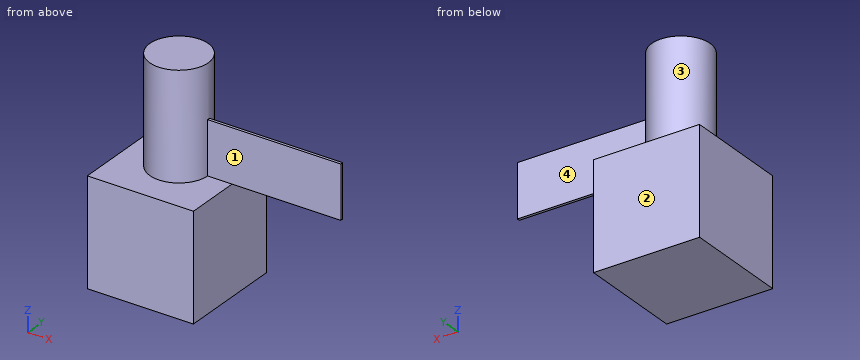
from build123d import *

# Parameters (mm, degrees)
F0_W     = 101.6
F0_H     = 101.6
F1_DEPTH = 101.6
F2_R     = 27.94
F3_DEPTH = 101.6
F5_W     = 156.614647
F5_H     = 2.673365
F6_DEPTH = 50.8


with BuildPart() as f1:
    # F0 (on Front) → F1 (new body)
    with BuildSketch(Plane.XZ):
        with Locations((-50.8, 50.8)):
            Rectangle(F0_W, F0_H)
    extrude(amount=F1_DEPTH)

    # F2 (on face) → F3 (join)
    with BuildSketch(Plane.XY.offset(101.6)):
        with Locations((-51.241014, -47.230963)):
            Circle(F2_R)
    extrude(amount=F3_DEPTH)

    # F5 (on face) → F6 (join)
    with BuildSketch(Plane.XY.offset(101.6)):
        with Locations((25.729626, -46.562624)):
            Rectangle(F5_W, F5_H)
    extrude(amount=F6_DEPTH)


solid = f1.part
Read the model definition and answer for the solid it produces. Units are mm, in the model's axes. Face numbers are marked on the shaded views. A direction names the side the tool comes from. Coordinates: 2 decimals unless noted, no trailing zeros. Write each loop counter-clockwise with the first axis right and the second up, starting at its lowest first coordinate (ties: lowest second). Pieces come first, ordered by that corner, then holes. Notation, with made-up numbers: (48.25, 6.5) -> (103.25, 6.5) arc R15 cw to (103.25, 31.5) -> close; hole circle Ø9 at (-1, -35). An arc over 180 degrees is marked (long way). Return JSON: item names as keys, results as strings.
(1) The part is cut by section A-A on y = -25. Give the vertices of the cut face in (x, z), then the cut area to 3 significant figures.
Answers below:
{"outline": "(-101.6, 0) -> (0, 0) -> (0, 101.6) -> (-34.32, 101.6) -> (-34.32, 203.2) -> (-68.17, 203.2) -> (-68.17, 101.6) -> (-101.6, 101.6) -> close", "area": "13,800 mm^2"}
(2) Each of these flat-tipped pins is pushed along its axis until it touches: P1, Ø5, axis at x = -22, y = -16, coming from the +Z side; P2, Ø8, axis at x = 72.5, y = -38, coming from the -Z side; P3, Ø1.3, axis at x = 25, y = -46.5, coming from the +Z side; P4, Ø8, axis at y = -73.5, z = 132, coming from the +X side. Where does it stop, or does it pass through?
Answers below:
{"P1": "z = 101.6", "P2": "through", "P3": "z = 152.4", "P4": "x = -34.37"}
(3) Consider line 1 along Y through (x, z) = (76, 103); line 2 along Z through (x, y) = (-41, -19.5); line 3 along X through (y, z) = (-86, 101). Determine where each line is inside the solid, lowest interval first. Write a range as from..to.
Answers below:
{"line 1": "-47.9..-45.23", "line 2": "0..101.6", "line 3": "-101.6..0"}
(4) Which of the six approach directions +Z, -Z, +X, -X, +Y, -Y give full straight-line access (tool end or side, diameter ignored) to the marked faces 1, 2, 3 and 4?
Answers below:
{"face 1": "+Z, +X, -Y", "face 2": "+Z, -Z, +X, -X, +Y", "face 3": "+Z", "face 4": "+Z, +X, +Y"}
(5) The part is cut by section C-C on z = 84.5. Give the vertices of the cut face in (x, y), then the cut area to 3 significant figures.
Answers below:
{"outline": "(-101.6, -101.6) -> (0, -101.6) -> (0, 0) -> (-101.6, 0) -> close", "area": "10,300 mm^2"}
(6) The part is cut by section B-B on x = 27. Give the vertices of the cut face in (y, z).
Answers below:
{"outline": "(-47.9, 101.6) -> (-45.23, 101.6) -> (-45.23, 152.4) -> (-47.9, 152.4) -> close"}
(7) The part is cut by section D-D on y = -68. Give the vertices of the cut face in (x, z).
Answers below:
{"outline": "(-101.6, 0) -> (0, 0) -> (0, 101.6) -> (-32.55, 101.6) -> (-32.55, 203.2) -> (-69.93, 203.2) -> (-69.93, 101.6) -> (-101.6, 101.6) -> close"}
